Verification items for the finished model (mm, model axes). A direction names the side the tool comes from. Round coordinates to 2 decimals unless told otherwise and drop trailing zeros. Write each loop counter-clockwise with the first axis right and the second up, starting at its lowest first coordinate (ties: lowest second). Pieces come first, ordered by that corner, then holes. Notation, with made-up numbers: M 7.5,86.5 L 26.5,86.5 A16 ccw 26.5,98.5 Z; hole C -12,-6 d8. An arc over 180 degrees is marked long. One line per item, written item: value. Start each with the question number.
Item 1: Thickness scan on probe 1 along Z at (x, y) = (0, -9.75); probe 2 along Z at (x, y) = (3, -3.25); probe 3 along Y at (x, z) = (-22, 20.5). Record the ranges inside material, lowest first. Write a range as from..to.
Item 2: Section check A-A, the plane x = 0. Record the cut outline in (y, z).
Item 3: Section check D-D, the plane y = -17. Record the cut outline in (x, z), then the cut area to 3 significant figures.
Item 4: Section check C-C, the plane y = -3.5. Record the cut outline in (x, z), then the cut area to 3 significant figures.
Item 5: Section check B-B, the plane z = 0. Record the cut outline in (x, y).
Item 6: Draft check along X on faces 3 (the face through (20, -20, 8)), 4 (the face through (-15.8, -10.1, -12.1)), 5 (the face through (31, -2.97, 9.76)). Enter one of: +X half, -X half, draft (parallel to the pull), parting line (faces both ways), or undercut.
Item 7: Tool access check on faces 1 (the face through (21, 0, -7)), 2 (the face through (-27, -5, 7)). Record the directions out of +Z, -Z, +X, -X, +Y, -Y that give a thin tool (end or side, any length) a straight path to the whole face; none if there is none.
Item 8: Gauge pin test, flat ends, axial feed: pin 1 (3 mm diameter, centred on x = -14, y = -16.5, fed in from +Z); pin 2 (2 mm diameter, centred on y = -8.5, z = 22.5, fed in from +X); pin 3 (10 mm diameter, centred on y = -6, z = 15, fed in from +X). Record the tip position at first contact, or that the pin passes through.
from build123d import *

# Parameters (mm, degrees)
F0_R     = 32.5
F1_DEPTH = 5
F2_R     = 27.5
F3_DEPTH = 15
F4_R     = 19.9
F5_DEPTH = 25
F6_SIZE  = 1


with BuildPart() as f1:
    # F0 (on Front) → F1 (new body)
    with BuildSketch(Plane.XZ):
        Circle(F0_R)
    extrude(amount=F1_DEPTH)

    # F2 (on face) → F3 (join)
    with BuildSketch(Plane.XZ.offset(5)):
        Circle(F2_R)
    extrude(amount=F3_DEPTH)

    # F4 (on face) → F5 (cut)
    with BuildSketch(Plane.XZ.offset(20)):
        Circle(F4_R)
    extrude(amount=-F5_DEPTH, mode=Mode.SUBTRACT)

    # F6
    f6_edges = [f1.edges().sort_by_distance(p)[0] for p in [
        (-32.5, 0, 0),
        (-27.5, -20, 0),
        (-19.9, -20, 0),
        (-19.9, 0, 0),
    ]]
    chamfer(f6_edges, length=F6_SIZE)


solid = f1.part
Response values:
1. probe 1: z = -27.5..-19.9, 19.9..27.5
1. probe 2: z = -32.36..-19.67, 19.67..32.36
1. probe 3: y = -5..0
2. outline: M -20,-26.5 L -19,-27.5 L -5,-27.5 L -5,-32.5 L -1,-32.5 L 0,-31.5 L 0,-20.9 L -1,-19.9 L -19,-19.9 L -20,-20.9 Z; M -20,20.9 L -19,19.9 L -1,19.9 L 0,20.9 L 0,31.5 L -1,32.5 L -5,32.5 L -5,27.5 L -19,27.5 L -20,26.5 Z
3. outline: C 0,0 d55; hole C 0,0 d39.8
3. area: 1,130 mm2
4. outline: C 0,0 d65; hole C 0,0 d39.8
4. area: 2,070 mm2
5. outline: M -32.5,-5 L -27.5,-5 L -27.5,-19 L -26.5,-20 L -20.9,-20 L -19.9,-19 L -19.9,-1 L -20.9,0 L -31.5,0 L -32.5,-1 Z; M 19.9,-19 L 20.9,-20 L 26.5,-20 L 27.5,-19 L 27.5,-5 L 32.5,-5 L 32.5,-1 L 31.5,0 L 20.9,0 L 19.9,-1 Z
6. face 3: draft
6. face 4: undercut
6. face 5: parting line
7. face 1: +Z, -Z, +X, -X, +Y
7. face 2: -Y
8. pin 1: stops at z = 24.49
8. pin 2: stops at x = 17.15
8. pin 3: stops at x = 30.89
